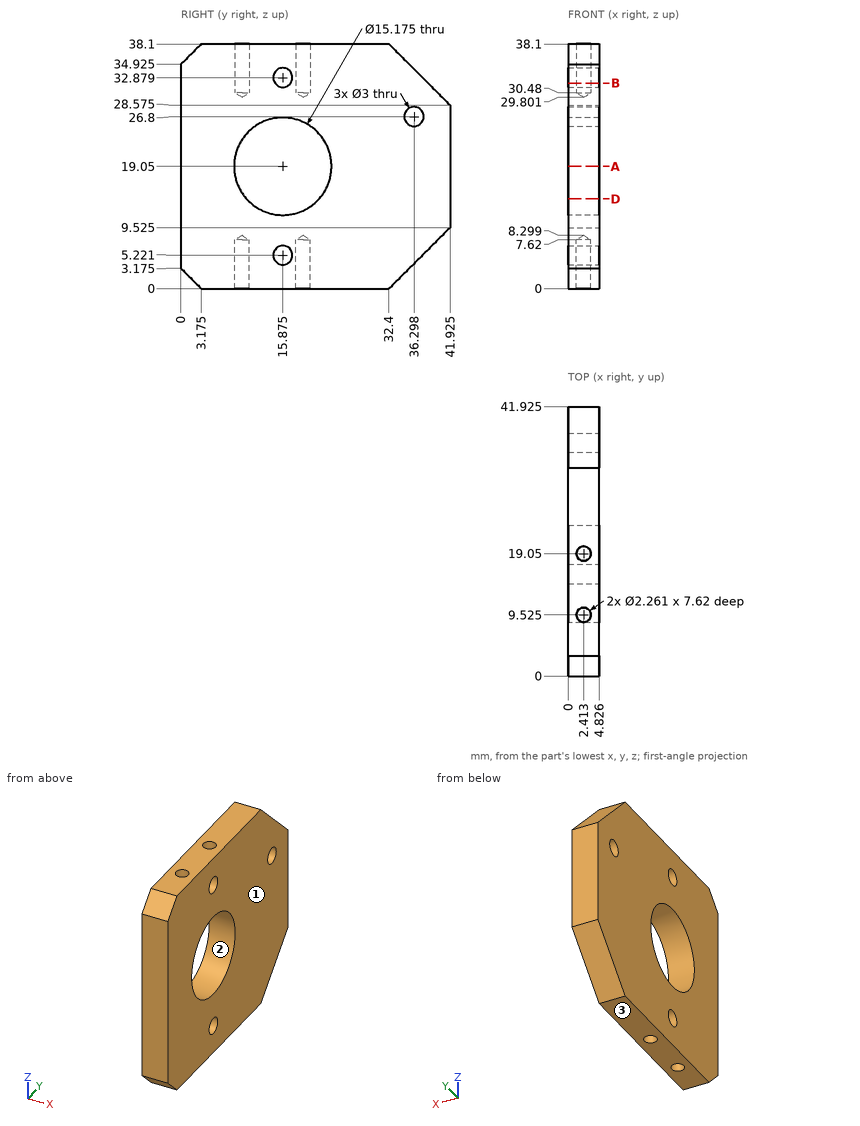
The drawing under review shows one solid part. Ordinate dimensions are in mm from its lowest x, y, z. Coordinates: 2 decimals unless noted, no trailing zeros. Write each loop counter-clockwise with the first axis right and the second up, starting at its lowest first coordinate (ties: lowest second). Pieces come first, ordered by that corner, then holes. Notation, with made-up numbers: (-37, -13) - (16, -13) arc R16 ccw to (16, 6) - close; hole circle Ø1 at (21, 4). An arc over 180 degrees is marked (long way). Use one line per item in the form item = value.
Q1. Consider section D-D (z = 14). Write out the cut boundary in (x, y) (1 decimal).
Taken from the geometry:
outline = (0, 0) - (4.8, 0) - (4.8, 10.2) - (0, 10.2) - close; (0, 21.5) - (4.8, 21.5) - (4.8, 41.9) - (0, 41.9) - close
Q2. The part is to be moulded in two halves that separate along Z. For the marked faces 1, 2 and 3, say which applies: +Z half, -Z half, draft (parallel to the pull), parting line (faces both ways), or undercut.
Taken from the geometry:
face_1 = draft
face_2 = undercut
face_3 = -Z half
Q3. Insertion check: pin 1 Ø1.8 at (x, y) = (2.413, 19.05) entering from +Z; pin 2 Ø1.4 at (x, y) = (2.413, 9.525) entering from +Z; pin 3 Ø1.4 at (x, y) = (2.413, 9.525) entering from -Z. Each pin has a flat end and moves straight along its axis. Give the tip position at first contact, or say it passes through.
Taken from the geometry:
pin_1 = 30.34
pin_2 = 30.22
pin_3 = 7.88
Q4. Consider section A-A (z = 19.05). Write out the cut boundary in (x, y) (1 decimal).
Taken from the geometry:
outline = (0, 0) - (4.8, 0) - (4.8, 8.3) - (0, 8.3) - close; (0, 23.5) - (4.8, 23.5) - (4.8, 41.9) - (0, 41.9) - close
Q5. For probe 1 along X at (y, z) = (19, 2); probe 2 along Z at (x, y) = (1.7, 15) (1 decimal); probe 3 along Y at (x, z) = (2.35, 26.8) (1 decimal), list the stretches that pass through material, from the lowest coordinate up.
Taken from the geometry:
probe_1 = 0 to 1.28, 3.54 to 4.83
probe_2 = 0 to 4, 6.4 to 11.5, 26.6 to 31.7, 34.1 to 38.1
probe_3 = 0 to 34.8, 37.8 to 41.9
Q6. Consider section B-B (z = 32). Count the separate pieces of the cut face and the enclosed holes in it, plus the area to 3 significant figures.
Taken from the geometry:
separate_pieces = 2
enclosed_holes = 2
area = 166 mm^2
